Can you work these out from the model? Positions are in its coordinate system, mm. A direction names the side the tool comes from. Round coordinates to 2 decimals unless told otherwise and drop trailing zeros. Order: outer loops, then holes, each group sorted by start corner. A loop starts at its lowest first (then second) coordinate and runs counter-clockwise, first axis right, second up.
from build123d import *

# Parameters (mm, degrees)
SKETCH1_W           = 10
SKETCH1_H           = 25.4
BOSS_EXTRUDE1_DEPTH = 2
SKETCH3_W           = 10
SKETCH3_H           = 3
BOSS_EXTRUDE3_DEPTH = 3
SKETCH4_W           = 10
SKETCH4_H           = 1.5
BOSS_EXTRUDE4_DEPTH = 15
SKETCH5_R           = 1.5
CUT_EXTRUDE1_DEPTH  = 14.974619852
FILLET2_R           = 1
FILLET4_RADIUS      = 0.75
FILLET4_LENGTH      = 10
FILLET5_R           = 1
FILLET6_R           = 1
FILLET7_R           = 1
FILLET8_START       = -1
FILLET8_DEPTH       = 5
FILLET9_START       = -1
FILLET9_DEPTH       = 4
FILLET10_R          = 1
FILLET11_R          = 1


with BuildPart() as part:
    # Sketch1 → Boss-Extrude1 (new body)
    with BuildSketch(Plane(origin=(0, 0, 0), x_dir=(1, 0, 0), z_dir=(0, 1, 0))):
        Rectangle(SKETCH1_W, SKETCH1_H)
    extrude(amount=BOSS_EXTRUDE1_DEPTH)

    # Sketch3 → Boss-Extrude3 (add)
    with BuildSketch(Plane(origin=(0, 2, 0), x_dir=(1, 0, 0), z_dir=(0, 1, 0))):
        with Locations((0, -8.2)):
            Rectangle(SKETCH3_W, SKETCH3_H)
    extrude(amount=BOSS_EXTRUDE3_DEPTH)

    # Sketch4 → Boss-Extrude4 (add)
    with BuildSketch(Plane(origin=(0, 0, 6.7), x_dir=(-1, 0, 0), z_dir=(0, 0, -1))):
        with Locations((0, 4.25)):
            Rectangle(SKETCH4_W, SKETCH4_H)
    extrude(amount=BOSS_EXTRUDE4_DEPTH)

    # Sketch5 → Cut-Extrude1 (cut, through all)
    with BuildSketch(Plane(origin=(0, 2, 0), x_dir=(1, 0, 0), z_dir=(0, 1, 0))):
        with Locations(Location((0, 10.2, 0), (0, 0, 270))):
            Circle(SKETCH5_R)
    extrude(amount=-CUT_EXTRUDE1_DEPTH, mode=Mode.SUBTRACT)

    # Fillet2
    fillet2_edges = [part.edges().sort_by_distance(p)[0] for p in [
        (0, 2, -11.7),
    ]]
    fillet(fillet2_edges, radius=FILLET2_R - 0.0001)  # a hair under: the kernel refuses the full size

    # Fillet4: full round fillet: the end face becomes a half cylinder, R = half its width
    fillet4_face = Plane((0, 4.25, -8.3), x_dir=(1, 0, 0), z_dir=(0, 0, -1))  # on the end face: x along it, z out of the body
    fillet4_slab = fillet4_face.offset(-FILLET4_RADIUS / 2) * Box(FILLET4_LENGTH, 2 * FILLET4_RADIUS, FILLET4_RADIUS, mode=Mode.PRIVATE)  # the body's end, R deep
    fillet4_round = Plane((0, 4.25, -7.55), x_dir=(0, 0, -1), z_dir=(1, 0, 0)) * Cylinder(FILLET4_RADIUS, FILLET4_LENGTH, mode=Mode.PRIVATE)  # its axis R under the face
    add(fillet4_slab - fillet4_round, mode=Mode.SUBTRACT)

    # Fillet5
    # the kernel refuses this fillet: 1 mm, written as the material it takes off along each edge
    with BuildSketch(Plane(origin=(7.5, 2, 12.7), x_dir=(0, -1, 0), z_dir=(-1, 0, 0))) as fillet5_piece_1:
        with BuildLine():
            CenterArc((FILLET5_R, -FILLET5_R), FILLET5_R, 90, 90)
            Line((0, -FILLET5_R), (0, 0))
            Line((0, 0), (FILLET5_R, 0))
        make_face()
    extrude(amount=15, mode=Mode.SUBTRACT)
    with BuildSketch(Plane(origin=(-5, 2, 15.2), x_dir=(1, 0, 0), z_dir=(0, 0, -1)), Plane(origin=(-5, 2, 9.7), x_dir=(1, 0, 0), z_dir=(0, 1, 0)), Plane(origin=(5, 2, 9.7), x_dir=(0, 0, -1), z_dir=(0, 1, 0))) as fillet5_piece_2:
        with BuildLine():
            CenterArc((FILLET5_R, FILLET5_R), FILLET5_R, 180, 90)
            Line((0, FILLET5_R), (0, 0))
            Line((0, 0), (FILLET5_R, 0))
        make_face()
    extrude(amount=5.5, mode=Mode.SUBTRACT)
    with BuildSketch(Plane(origin=(5, 5, -10.05), x_dir=(0, -1, 0), z_dir=(0, 0, 1))) as fillet5_piece_3:
        with BuildLine():
            CenterArc((FILLET5_R, -FILLET5_R), FILLET5_R, 90, 90)
            Line((0, -FILLET5_R), (0, 0))
            Line((0, 0), (FILLET5_R, 0))
        make_face()
    extrude(amount=22.25, mode=Mode.SUBTRACT)
    with BuildSketch(Plane(origin=(5, 2, 9.7), x_dir=(0, -1, 0), z_dir=(0, 0, 1))) as fillet5_piece_4:
        with BuildLine():
            CenterArc((FILLET5_R, -FILLET5_R), FILLET5_R, 90, 90)
            Line((0, -FILLET5_R), (0, 0))
            Line((0, 0), (FILLET5_R, 0))
        make_face()
    extrude(amount=5.5, mode=Mode.SUBTRACT)
    with BuildSketch(Plane(origin=(-5, 5, 12.2), x_dir=(1, 0, 0), z_dir=(0, 0, -1))) as fillet5_piece_5:
        with BuildLine():
            CenterArc((FILLET5_R, FILLET5_R), FILLET5_R, 180, 90)
            Line((0, FILLET5_R), (0, 0))
            Line((0, 0), (FILLET5_R, 0))
        make_face()
    extrude(amount=22.25, mode=Mode.SUBTRACT)
    with BuildSketch(Plane(origin=(-5, 2, 15.2), x_dir=(1, 0, 0), z_dir=(0, 0, -1))) as fillet5_piece_6a_section:
        with BuildLine():
            CenterArc((FILLET5_R, FILLET5_R), FILLET5_R, 180, 90)
            Line((0, FILLET5_R), (0, 0))
            Line((0, 0), (FILLET5_R, 0))
        make_face()
    fillet5_piece_6a = extrude(amount=8, mode=Mode.PRIVATE)
    fillet5_piece_6a = split(fillet5_piece_6a, bisect_by=Plane(origin=(-5, 2, 9.7), z_dir=(0, 0, -1)), keep=Keep.TOP, mode=Mode.PRIVATE)
    with BuildSketch(Plane(origin=(-5, -0.5, 9.7), x_dir=(1, 0, 0), z_dir=(0, 1, 0))) as fillet5_piece_6b_section:
        with BuildLine():
            CenterArc((FILLET5_R, FILLET5_R), FILLET5_R, 180, 90)
            Line((0, FILLET5_R), (0, 0))
            Line((0, 0), (FILLET5_R, 0))
        make_face()
    fillet5_piece_6b = extrude(amount=8, mode=Mode.PRIVATE)
    fillet5_piece_6b = split(fillet5_piece_6b, bisect_by=Plane(origin=(-5, 2, 9.7), z_dir=(0, -1, 0)), keep=Keep.TOP, mode=Mode.PRIVATE)
    fillet5_piece_6 = fillet5_piece_6a & fillet5_piece_6b
    add(fillet5_piece_6, mode=Mode.SUBTRACT)
    with BuildSketch(Plane(origin=(5, -0.5, 9.7), x_dir=(0, 0, -1), z_dir=(0, 1, 0))) as fillet5_piece_7a_section:
        with BuildLine():
            CenterArc((FILLET5_R, FILLET5_R), FILLET5_R, 180, 90)
            Line((0, FILLET5_R), (0, 0))
            Line((0, 0), (FILLET5_R, 0))
        make_face()
    fillet5_piece_7a = extrude(amount=8, mode=Mode.PRIVATE)
    fillet5_piece_7a = split(fillet5_piece_7a, bisect_by=Plane(origin=(5, 2, 9.7), z_dir=(0, -1, 0)), keep=Keep.TOP, mode=Mode.PRIVATE)
    with BuildSketch(Plane(origin=(5, 2, 7.2), x_dir=(0, -1, 0), z_dir=(0, 0, 1))) as fillet5_piece_7b_section:
        with BuildLine():
            CenterArc((FILLET5_R, -FILLET5_R), FILLET5_R, 90, 90)
            Line((0, -FILLET5_R), (0, 0))
            Line((0, 0), (FILLET5_R, 0))
        make_face()
    fillet5_piece_7b = extrude(amount=8, mode=Mode.PRIVATE)
    fillet5_piece_7b = split(fillet5_piece_7b, bisect_by=Plane(origin=(5, 2, 9.7), z_dir=(0, 0, -1)), keep=Keep.TOP, mode=Mode.PRIVATE)
    fillet5_piece_7 = fillet5_piece_7a & fillet5_piece_7b
    add(fillet5_piece_7, mode=Mode.SUBTRACT)

    # Fillet6
    fillet6_edges = [part.edges().sort_by_distance(p)[0] for p in [
        (-5, 2, -3),
    ]]
    fillet(fillet6_edges, radius=FILLET6_R)

    # Fillet7
    fillet7_edges = [part.edges().sort_by_distance(p)[0] for p in [
        (5, 2, -3),
    ]]
    fillet(fillet7_edges, radius=FILLET7_R)

    # Fillet8: read off the stored shape, not the designer's step
    # Fillet8 outline → Fillet8 (cut)
    with BuildSketch(Plane(origin=(0, 0, 0), x_dir=(1, 0, 0), z_dir=(0, 1, 0)).offset(FILLET8_START)):
        with BuildLine():
            Line((-5, 12.7), (-5, 11.7))
            add(Edge.make_bspline(
                [(-5, 11.7), (-5, 12.7), (-4, 12.7)],
                knots=[0, 0, 0, 1, 1, 1], degree=2, weights=[1, 0.707106781, 1]))
            Line((-4, 12.7), (-5, 12.7))
        make_face()
    extrude(amount=FILLET8_DEPTH, mode=Mode.SUBTRACT)

    # Fillet9: read off the stored shape, not the designer's step
    # Fillet9 outline → Fillet9 (cut)
    with BuildSketch(Plane(origin=(0, 0, 0), x_dir=(1, 0, 0), z_dir=(0, 1, 0)).offset(FILLET9_START)):
        with BuildLine():
            Line((5, 12.7), (4, 12.7))
            add(Edge.make_bspline(
                [(4, 12.7), (5, 12.7), (5, 11.7)],
                knots=[0, 0, 0, 1, 1, 1], degree=2, weights=[1, 0.707106781, 1]))
            Line((5, 11.7), (5, 12.7))
        make_face()
    extrude(amount=FILLET9_DEPTH, mode=Mode.SUBTRACT)

    # Fillet10
    # the kernel refuses this fillet: 1 mm, written as the material it takes off along each edge
    with BuildSketch(Plane(origin=(-4, 1, 11.7), x_dir=(0, 0, 1), z_dir=(-1, 0, 0))) as fillet10_piece_1_section:
        Polygon((0, 0), (FILLET10_R, 0), (FILLET10_R, FILLET10_R), (0, FILLET10_R), align=None)
    fillet10_piece_1 = extrude(amount=FILLET10_R, mode=Mode.PRIVATE)
    fillet10_piece_1 = fillet10_piece_1 - Plane(origin=(-4, 1, 11.7), x_dir=(0, -0.7071067811865475, -0.7071067811865475), z_dir=(-1, 0, 0)) * Sphere(FILLET10_R, mode=Mode.PRIVATE)
    add(fillet10_piece_1, mode=Mode.SUBTRACT)
    with BuildSketch(Plane(origin=(-5, -2.5, 12.7), x_dir=(0, 0, -1), z_dir=(0, 1, 0))) as fillet10_piece_2:
        with BuildLine():
            CenterArc((FILLET10_R, -FILLET10_R), FILLET10_R, 90, 90)
            Line((0, -FILLET10_R), (0, 0))
            Line((0, 0), (FILLET10_R, 0))
        make_face()
    extrude(amount=3.5, mode=Mode.SUBTRACT)

    # Fillet11
    # the kernel refuses this fillet: 1 mm, written as the material it takes off along each edge
    with BuildSketch(Plane(origin=(4, 1, 11.7), x_dir=(0, 0, 1), z_dir=(1, 0, 0))) as fillet11_piece_1_section:
        Polygon((0, 0), (FILLET11_R, 0), (FILLET11_R, -FILLET11_R), (0, -FILLET11_R), align=None)
    fillet11_piece_1 = extrude(amount=FILLET11_R, mode=Mode.PRIVATE)
    fillet11_piece_1 = fillet11_piece_1 - Plane(origin=(4, 1, 11.7), x_dir=(0, -0.7071067811865475, -0.7071067811865475), z_dir=(1, 0, 0)) * Sphere(FILLET11_R, mode=Mode.PRIVATE)
    add(fillet11_piece_1, mode=Mode.SUBTRACT)
    with BuildSketch(Plane(origin=(5, -2.5, 12.7), x_dir=(0, 0, -1), z_dir=(0, 1, 0))) as fillet11_piece_2:
        with BuildLine():
            CenterArc((FILLET11_R, FILLET11_R), FILLET11_R, 180, 90)
            Line((0, FILLET11_R), (0, 0))
            Line((0, 0), (FILLET11_R, 0))
        make_face()
    extrude(amount=3.5, mode=Mode.SUBTRACT)


solid = part.part
(1) I'm going to push flat-ended pins straight in: pin 1 Ø0.9 at (x, y) = (1, 4) entering from +Z; pin 2 Ø2 at (y, z) = (2, -5) entering from -X; pin 3 Ø0.6 at (x, z) = (-0.5, 10.5) entering from +Y. Where does each tip first touch, or does it pass through?
(2) If we mould it in two halves opening along X, with no side actions, what happens to faces 1 (the face through (4.715, 4.699, 0.574)), 2 (the face through (-4.715, 1.699, 10.554)), 3 (the face through (0, 0, 0)), 4 (the face through (-0.575, 0.507, -8.814))? For each: pulls with the +X half, pulls with the -X half, needs draft (parallel to the pull), parting line crosses it, or undercut.
(3) I want a section at C-C, the plane z = -10.2. List the corners of the cut face in (x, y) for me.
(4) On a 3-axis mill with a long thin cutter (end or side, diameter ignored), from which of +Z, -Z, +X, -X, +Y, -Y can I reach the whole of each face in a straight line? I mean faces 5 (the face through (4.715, 1.699, 10.512)), 6 (the face through (0, 3.5, 0)), 7 (the face through (-4.699, 1.715, -3.136)). Say none if no direction works.
(5) I want a section at B-B, the plane z = -1.25. List the corners of the cut face in (x, y) for me.
(6) Please list where these lines run through material, in increasing order: probe 1 along X at (y, z) = (0.8, -10.2); probe 2 along Y at (x, z) = (-1.5, -7); probe 3 along Y at (x, z) = (-1, 11.5).
(7) I want a section at D-D, the plane y = 4.25. List the corners of the cut face in (x, z) for me.
Ans:
1. pin 1: stops at z = 9.7
1. pin 2: stops at x = -5
1. pin 3: stops at y = 2
2. face 1: pulls with the +X half
2. face 2: pulls with the -X half
2. face 3: needs draft
2. face 4: undercut
3. outline: (-5, 0) - (-1.5, 0) - (-1.5, 1) arc R1 ccw to (-2.5, 2) - (-4, 2) arc R1 ccw to (-5, 1) - close; (1.5, 0) - (5, 0) - (5, 1) arc R1 ccw to (4, 2) - (2.5, 2) arc R1 ccw to (1.5, 1) - close
4. face 5: +Z, +X, +Y
4. face 6: -Z, +X, -X
4. face 7: -Z, -X
5. outline: (-5, 0) - (5, 0) - (5, 1) arc R1 ccw to (4, 2) - (-4, 2) arc R1 ccw to (-5, 1) - close; (-5, 3.5) - (5, 3.5) - (5, 4) arc R1 ccw to (4, 5) - (-4, 5) arc R1 ccw to (-5, 4) - close
6. probe 1: x = -5 to -1.5, 1.5 to 5
6. probe 2: y = 0 to 2, 3.5 to 5
6. probe 3: y = 0 to 2
7. outline: (-4.97, -8.3) - (4.97, -8.3) - (4.97, 8.95) arc R1 ccw to (4, 9.7) - (-4, 9.7) arc R1 ccw to (-4.97, 8.95) - close
